```python
from build123d import *

# Parameters (mm, degrees)
SKETCH2_W               = 52
SKETCH2_H               = 58
SKETCH2_W_2             = 26
SKETCH2_H_2             = 26
BOSS_EXTRUDE1_DEPTH     = 5
SKETCH3_W               = 4.8
SKETCH3_H               = 4.8
BOSS_EXTRUDE2_DEPTH     = 15
M4_CLEARANCE_HOLE1_D    = 4.5
MIRROR2_COPY_1_SKETCH_W = 4.8
MIRROR2_COPY_1_SKETCH_H = 4.8
MIRROR2_COPY_1_DEPTH    = 15
MIRROR2_COPY_2_D        = 4.5
SKETCH7_W               = 6
SKETCH7_H               = 15
CUT_EXTRUDE1_DEPTH      = 44.783558558
CHAMFER1_SIZE           = 2
BOSS_EXTRUDE4_DEPTH     = 2.5
CHAMFER2_SIZE           = 4
FILLET1_R               = 1


with BuildPart() as part:
    # Sketch2 → Boss-Extrude1 (new body)
    with BuildSketch(Plane(origin=(0, 0, 0), x_dir=(0, 0, -1), z_dir=(1, 0, 0))):
        Rectangle(SKETCH2_W, SKETCH2_H)
        Rectangle(SKETCH2_W_2, SKETCH2_H_2, mode=Mode.SUBTRACT)
    extrude(amount=BOSS_EXTRUDE1_DEPTH)

    # Sketch3 → Boss-Extrude2 (add)
    with BuildSketch(Plane(origin=(5, 0, 0), x_dir=(0, 0, -1), z_dir=(1, 0, 0))):
        with Locations((-23.6, 26.6)):
            Rectangle(SKETCH3_W, SKETCH3_H)
    boss_extrude2 = extrude(amount=BOSS_EXTRUDE2_DEPTH)

    # M4 Clearance Hole1 (through all)
    with Locations(Plane(origin=(0, 25, 22), x_dir=(0, 0, -1), z_dir=(-1, 0, 0))):
        with Locations((0, 0)):
            m4_clearance_hole1 = Hole(M4_CLEARANCE_HOLE1_D / 2)

    # Mirror1: Boss-Extrude2, M4 Clearance Hole1 across plane
    add(boss_extrude2.mirror(Plane.XY))
    add(m4_clearance_hole1.mirror(Plane.XY), mode=Mode.SUBTRACT)

    # Mirror2: Boss-Extrude2, M4 Clearance Hole1 across plane
    add(boss_extrude2.mirror(Plane.ZX))
    add(m4_clearance_hole1.mirror(Plane.ZX), mode=Mode.SUBTRACT)

    # Mirror2 copy 1 sketch → Mirror2 copy 1 (add)
    with BuildSketch(Plane(origin=(5, 0, 0), x_dir=(0, 0, 1), z_dir=(1, 0, 0))):
        with Locations((-23.6, 26.6)):
            Rectangle(MIRROR2_COPY_1_SKETCH_W, MIRROR2_COPY_1_SKETCH_H)
    extrude(amount=MIRROR2_COPY_1_DEPTH)

    # Mirror2 copy 2 (through all)
    with Locations(Plane(origin=(0, -25, -22), x_dir=(0, 0, 1), z_dir=(-1, 0, 0))):
        with Locations((0, 0)):
            Hole(MIRROR2_COPY_2_D / 2)

    # Sketch7 → Cut-Extrude1 (cut, through all)
    with BuildSketch(Plane.ZY):
        with Locations((-23, 13.5)):
            Rectangle(SKETCH7_W, SKETCH7_H)
    cut_extrude1 = extrude(amount=-CUT_EXTRUDE1_DEPTH, mode=Mode.SUBTRACT)

    # Mirror3: Cut-Extrude1 across plane
    add(cut_extrude1.mirror(Plane.ZX), mode=Mode.SUBTRACT)

    # Chamfer1
    chamfer1_edges = [part.edges().sort_by_distance(p)[0] for p in [
        (2.5, 21, -20),
        (2.5, -21, -20),
    ]]
    chamfer(chamfer1_edges, length=CHAMFER1_SIZE)

    # Sketch9 → Boss-Extrude4 (add)
    with BuildSketch(Plane.XZ.offset(29)):
        Polygon((0, 26), (0, -26), (20, -26), (20, -21.2), (5, -21.2), (5, 21.2), (20, 21.2), (20, 26), align=None)
    extrude(amount=BOSS_EXTRUDE4_DEPTH)

    # Chamfer2
    chamfer2_edges = [part.edges().sort_by_distance(p)[0] for p in [
        (2.5, 6, -26),
        (2.5, -6, -26),
    ]]
    chamfer(chamfer2_edges, length=CHAMFER2_SIZE)

    # Fillet1
    fillet1_edges = [part.edges().sort_by_distance(p)[0] for p in [
        (0, 25, -26),
        (0, 12.5, -20),
        (0, -12.5, -20),
        (0, -21, -24),
        (0, 21, -24),
        (0, -20, -21),
        (0, 20, -21),
        (0, -31.5, 0),
        (0, 0, -26),
        (0, 6, -21),
        (0, -6, -21),
        (0, -4, -24),
        (0, 4, -24),
        (0, 29, 0),
        (0, -26.25, -26),
        (0, -1.25, 26),
    ]]
    fillet(fillet1_edges, radius=FILLET1_R)


solid = part.part
```
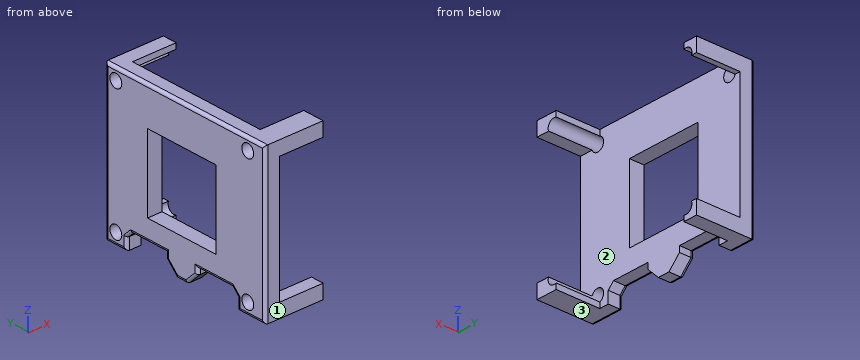
Here's how the part is built. I have some questions about the finished solid (model axes, mm). Face numbers are marked on the shaded views. Coordinates: 2 decimals unless noted, no trailing zeros. Order: outer loops, then holes, each group sorted by start corner. A loop starts at its lowest first (then second) coordinate and runs counter-clockwise, first axis right, second up. Notation, with made-up numbers: (58, 8) -> (116, 8) arc R22 ccw to (116, 27) -> close; hole circle Ø5 at (74, 9.5). An arc over 180 degrees is marked (long way). Return JSON: item names as keys, results as strings.
1) If we section it at C-C on y = 25: List the corners of the cut face in (x, z) for me, plus the area to 3 significant figures.
Conclusion:
{"outline": "(0, -25) arc R1 ccw to (1, -26) -> (20, -26) -> (20, -24.25) -> (0, -24.25) -> close; (0, -19.75) -> (5, -19.75) -> (5, 19.75) -> (0, 19.75) -> close; (0, 24.25) -> (20, 24.25) -> (20, 26) -> (1, 26) arc R1 ccw to (0, 25) -> close", "area": "267 mm²"}
2) If I drill on probe 1 along Z at (x, y) = (14, -25); probe 2 along Z at (x, y) = (4, -25); probe 3 along Y at (x, z) = (3.75, -9), over which ranges is the centre line in solid material (lowest first)?
Conclusion:
{"probe 1": "z = -26 to -24.25, 24.25 to 26", "probe 2": "z = -26 to -24.25, -19.75 to 19.75, 24.25 to 26", "probe 3": "y = -31.5 to -13, 13 to 29"}
3) Thinking about a two-plate mould opening in Y: for the marked faces 1, 2 and 3, which applies, +Y half, -Y half, draft (parallel to the pull), parting line (faces both ways), or undercut?
Conclusion:
{"face 1": "-Y half", "face 2": "undercut", "face 3": "draft"}
4) If we section it at B-B on x = 3.5: List the corners of the cut face in (y, z) for me.
Conclusion:
{"outline": "(-31.5, -26) -> (-21, -26) -> (-21, -22) -> (-19, -20) -> (-6, -20) -> (-6, -22) -> (-2, -26) -> (2, -26) -> (6, -22) -> (6, -20) -> (19, -20) -> (21, -22) -> (21, -26) -> (29, -26) -> (29, 26) -> (-31.5, 26) -> close; hole circle Ø4.5 at (-25, -22); hole circle Ø4.5 at (-25, 22); hole (-13, -13) -> (13, -13) -> (13, 13) -> (-13, 13) -> close; hole circle Ø4.5 at (25, -22); hole circle Ø4.5 at (25, 22)"}
5) I'm going to push flat-ended pins straight in: P1, Ø6, axis at y = -24.5, z = 19, coming from the +X side; P2, Ø2, axis at x = 3.5, y = 12, coming from the -Z side; P3, Ø3, axis at x = 3, y = -6, coming from the -Z side. Where does each tip first touch, or does it pass through?
Conclusion:
{"P1": "stops at x = 5", "P2": "stops at z = -20", "P3": "stops at z = -23.5"}
6) If we section it at A-A on z = 22: List the corners of the cut face in (x, y) for me.
Conclusion:
{"outline": "(0, -30.5) arc R1 ccw to (1, -31.5) -> (20, -31.5) -> (20, -27.25) -> (0, -27.25) -> close; (0, -22.75) -> (5, -22.75) -> (5, 22.75) -> (0, 22.75) -> close; (0, 27.25) -> (20, 27.25) -> (20, 29) -> (1, 29) arc R1 ccw to (0, 28) -> close"}
7) If we section it at D-D on z = -1.5: List the corners of the cut face in (x, y) for me, plus the area to 3 significant figures.
Conclusion:
{"outline": "(0, -30.5) arc R1 ccw to (1, -31.5) -> (5, -31.5) -> (5, -13) -> (0, -13) -> close; (0, 13) -> (5, 13) -> (5, 29) -> (1, 29) arc R1 ccw to (0, 28) -> close", "area": "172 mm²"}
